Could you check a few things on this model? Use its own coordinates, in mm. Face numbers are marked on the shaded views. Round coordinates to 2 decimals unless told otherwise and drop trailing zeros. Order: outer loops, then holes, each group sorted by start corner. A loop starts at its lowest first (then second) coordinate and runs counter-clockwise, first axis right, second up. Notation, with made-up numbers: (-2.75, -7.5) - (14.25, -7.5) arc R10 cw to (14.25, -0.5) - close; hole circle Ø5 at (-9, 28). An arc over 180 degrees is marked (long way). Return JSON: item names as keys, results as strings. Group by question number.
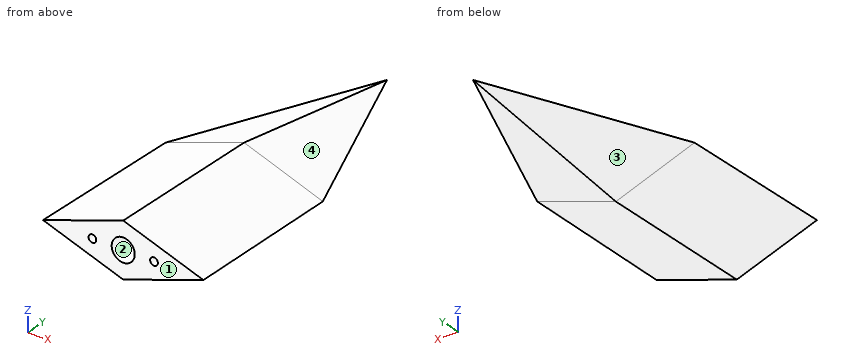
from build123d import *

# Parameters (mm, degrees)
BOSS_EXTRUDE1_DEPTH      = 11.1125
BOSS_EXTRUDE1_DEPTH_BACK = 11.1125
SKETCH5_W                = 109.877468776
SKETCH5_H                = 283.051122129
CUT_EXTRUDE2_DEPTH       = 1193.492852366
SKETCH6_W                = 149.121482991
SKETCH6_H                = 108.921761737
CUT_EXTRUDE3_DEPTH       = 1175.662940665
SKETCH7_R                = 4.7625
CUT_EXTRUDE4_DEPTH       = 635
CUT_EXTRUDE8_DEPTH       = 1195.766301895
CUT_EXTRUDE8_DEPTH_BACK  = 1195.766301895
SKETCH8_W                = 149.774750394
SKETCH8_H                = 148.832770831
SKETCH8_H_2              = 142.875
SKETCH17_R               = 1.5875
CUT_EXTRUDE15_DEPTH      = 12.7


with BuildPart() as part:
    # Sketch1 → Boss-Extrude1 (new, two sides: drawn at the far end of the back side and taken through both)
    with BuildSketch(Plane.XY.offset(-BOSS_EXTRUDE1_DEPTH_BACK)):
        Polygon((142.42123069, 465.168027231), (219.716026672, 465.168027231), (213.502471629, 1096.967634552), (181.068628681, 1174.337215652), (148.634785732, 1096.967634552), align=None)
    extrude(amount=BOSS_EXTRUDE1_DEPTH + BOSS_EXTRUDE1_DEPTH_BACK)

    # Sketch2 → Cut-Loft1 section 0
    with BuildSketch(Plane.XZ.offset(-465.168027231)):
        with BuildLine():
            Line((142.42123069, 0), (181.068628681, 11.1125))
            Line((181.068628681, 11.1125), (219.716026672, 0))
            Line((219.716026672, 0), (222.70513775, 0))
            Line((222.70513775, 0), (222.70513775, 15.258366339))
            Line((222.70513775, 15.258366339), (137.848628215, 15.258366339))
            Line((137.848628215, 15.258366339), (137.848628215, 0))
            Line((137.848628215, 0), (142.42123069, 0))
        make_face()
    # Sketch3 → Cut-Loft1 section 1
    with BuildSketch(Plane(origin=(0, 1096.967634552, 0), x_dir=(1, 0, 0), z_dir=(0, 1, 0))):
        with BuildLine():
            Line((213.502471629, 0), (181.068628681, -11.1125))
            Line((181.068628681, -11.1125), (148.634785732, 0))
            Line((148.634785732, 0), (137.848628215, 0))
            Line((137.848628215, 0), (137.848628215, -15.258366339))
            Line((137.848628215, -15.258366339), (222.70513775, -15.258366339))
            Line((222.70513775, -15.258366339), (222.70513775, 0))
            Line((222.70513775, 0), (213.502471629, 0))
        make_face()
    cut_loft1 = loft(mode=Mode.SUBTRACT)

    # Mirror1: Cut-Loft1 across plane
    add(cut_loft1.mirror(Plane.XY), mode=Mode.SUBTRACT)

    # Sketch5 → Cut-Extrude2 (cut, through all)
    with BuildSketch(Plane(origin=(-32.103098407, 13.457832356, 93.698704331), x_dir=(0.9470206004067627, 0.045661094409327196, 0.31791043842968925), z_dir=(-0.3211728232668741, 0.1346377834927197, 0.937401026696127))):
        with Locations((219.349244299, 1139.303724701)):
            Rectangle(SKETCH5_W, SKETCH5_H)
    cut_extrude2 = extrude(amount=CUT_EXTRUDE2_DEPTH, mode=Mode.SUBTRACT)

    # Sketch6 → Cut-Extrude3 (cut, through all)
    with BuildSketch(Plane(origin=(69.458274406, 29.117370568, 202.726547902), x_dir=(0.9470206004067623, -0.045661094409327495, -0.31791043842969063), z_dir=(0.3211728232668754, 0.13463778349272, 0.9374010266961263))):
        with Locations((131.752816965, 1118.922251835)):
            Rectangle(SKETCH6_W, SKETCH6_H)
    cut_extrude3 = extrude(amount=CUT_EXTRUDE3_DEPTH, mode=Mode.SUBTRACT)

    # Mirror2: Cut-Extrude2, Cut-Extrude3 across plane
    add(cut_extrude2.mirror(Plane.XY), mode=Mode.SUBTRACT)
    add(cut_extrude3.mirror(Plane.XY), mode=Mode.SUBTRACT)

    # Sketch7 → Cut-Extrude4 (cut)
    with BuildSketch(Plane.XZ.offset(-465.168027231)):
        with Locations(Location((181.068628681, 0, 0), (0, 0, 270))):
            Circle(SKETCH7_R)
    extrude(amount=-CUT_EXTRUDE4_DEPTH, mode=Mode.SUBTRACT)

    # Sketch8 → Cut-Extrude8 (cut, two sides: drawn at the far end of the back side and taken through both)
    with BuildSketch(Plane.XY.offset(-CUT_EXTRUDE8_DEPTH_BACK)):
        with Locations((180.5976389, 528.420830237)):
            Rectangle(SKETCH8_W, SKETCH8_H)
        with Locations((180.5976389, 674.274715652)):
            Rectangle(SKETCH8_W, SKETCH8_H_2)
        with Locations((180.5976389, 817.149715652)):
            Rectangle(SKETCH8_W, SKETCH8_H_2)
        with Locations((180.5976389, 960.024715652)):
            Rectangle(SKETCH8_W, SKETCH8_H_2)
    extrude(amount=CUT_EXTRUDE8_DEPTH + CUT_EXTRUDE8_DEPTH_BACK, mode=Mode.SUBTRACT)

    # Sketch17 → Cut-Extrude15 (cut)
    with BuildSketch(Plane.XZ.offset(-1031.462215652)):
        with Locations(Location((168.368628681, 0, 0), (0, 0, 270))):
            Circle(SKETCH17_R)
        with Locations(Location((193.768628681, 0, 0), (0, 0, 270))):
            Circle(SKETCH17_R)
    extrude(amount=-CUT_EXTRUDE15_DEPTH, mode=Mode.SUBTRACT)


solid = part.part
1) I want a section at A-A, the plane y = 1135. List the corners of the cut face in (x, z) for me, plus the area to 3 significant figures.
2) Will these pins go through, and if not, where does the flat tip stop? pin 1 (1 mm diameter, centred on x = 193, z = 0.5, fed in from -Y); pin 2 (10 mm diameter, centred on x = 197.5, y = 1099.5, fed in from +Z); pin 3 (2.5 mm diameter, centred on x = 193.77, z = 0, fed in from +Y).
3) We'd pull the mould along X, two halves only. Please class the marked faces 1, 2, 3 and 4: +X half, -X half, draft (parallel to the pull), parting line (faces both ways), or undercut.
4) I want a section at B-B, the plane y = 1113. List the corners of the cut face in (x, z) for me, plus the area to 3 significant figures.
5) If I drill on line 1 along Z through (x, y) = (180, 1046.5); line 2 along Z through (x, y) = (178, 1133); line 3 along Z through (x, y) = (177, 1046), over which ranges is the centre line in solid material (lowest first)? Write a range as from..to.
Outcome:
{
 "1": {"outline": "(164.58, 0) - (181.07, -5.65) - (197.56, 0) - (181.07, 5.65) - close", "area": "186 mm^2"},
 "2": {"pin 1": "y = 1044.16", "pin 2": "z = 6.98", "pin 3": "y = 1147.02"},
 "3": {"face 1": "draft", "face 2": "undercut", "face 3": "-X half", "face 4": "+X half"},
 "4": {"outline": "(155.36, 0) - (181.07, -8.81) - (206.78, 0) - (181.07, 8.81) - close", "area": "453 mm^2"},
 "5": {"line 1": "-10.75..-4.64, 4.64..10.75", "line 2": "-4.89..4.89", "line 3": "-9.74..-2.48, 2.48..9.74"}
}
